Read the model definition and answer for the solid it produces. Units are mm, in the model's axes. Round coordinates to 2 decimals unless told otherwise and drop trailing zeros. Loops run counter-clockwise (first coordinate to the right, second up) from the corner with the lowest first, then second, coordinate; pieces in that order, holes last. Notation, with made-up numbers: (87.5, -25.5) -> (141.5, -25.5) arc R13 ccw to (141.5, -12.5) -> close; hole circle Ø5 at (24, 48.5). An arc over 180 degrees is marked (long way). Put each result on its own line as item: value.
from build123d import *

# Parameters (mm, degrees)
SKETCH1_W                     = 735.584
SKETCH1_H                     = 38.1
WOOD_BLOCK_DEPTH              = 19.05
SKETCH2_R                     = 7.9756
INNER_BORE_DEPTH              = 737.816349952
SKETCH3_R                     = 6.3881
MOUTHPIECE_THROUGH_HOLE_DEPTH = 737.816349952
SKETCH5_R                     = 8.128
COUNTERBORE_DEPTH             = 8.89
SKETCH4_OUTSIDE_W             = 187.464
SKETCH4_OUTSIDE_H             = 168.414
SKETCH4_OUTSIDE_R             = 14.2875
OUTER_DIAMETER_DEPTH          = 737.816350054


with BuildPart() as part:
    # Sketch1 → wood block (new body)
    with BuildSketch(Plane(origin=(0, 0, 0), x_dir=(1, 0, 0), z_dir=(0, 1, 0))):
        with Locations((367.792, 19.05)):
            Rectangle(SKETCH1_W, SKETCH1_H)
    extrude(amount=WOOD_BLOCK_DEPTH)

    # Sketch2 → inner bore (cut, through all)
    with BuildSketch(Plane(origin=(735.584, 0, 0), x_dir=(0, 0, -1), z_dir=(1, 0, 0))):
        with Locations((19.05, 19.05)):
            Circle(SKETCH2_R)
    extrude(amount=-INNER_BORE_DEPTH, mode=Mode.SUBTRACT)

    # Sketch3 → mouthpiece through hole (cut, through all)
    with BuildSketch(Plane(origin=(0, 0, 0), x_dir=(1, 0, 0), z_dir=(0, 1, 0))):
        with Locations(Location((22.225, 19.05, 0), (0, 0, 90))):
            Circle(SKETCH3_R)
    extrude(amount=MOUTHPIECE_THROUGH_HOLE_DEPTH, mode=Mode.SUBTRACT)

    # Sketch5 → counterbore (cut)
    with BuildSketch(Plane.XZ):
        with Locations(Location((22.225, -19.05, 0), (0, 0, 270))):
            Circle(SKETCH5_R)
        with Locations(Location((713.359, -19.05, 0), (0, 0, 90))):
            Circle(SKETCH5_R)
    extrude(amount=-COUNTERBORE_DEPTH, mode=Mode.SUBTRACT)

    # Sketch4 outside → outer diameter (cut, through all)
    with BuildSketch(Plane.ZY):
        with Locations((-19.05, 9.525)):
            Rectangle(SKETCH4_OUTSIDE_W, SKETCH4_OUTSIDE_H)
        with Locations((-19.05, 19.05)):
            Circle(SKETCH4_OUTSIDE_R, mode=Mode.SUBTRACT)
    extrude(amount=-OUTER_DIAMETER_DEPTH, mode=Mode.SUBTRACT)


solid = part.part
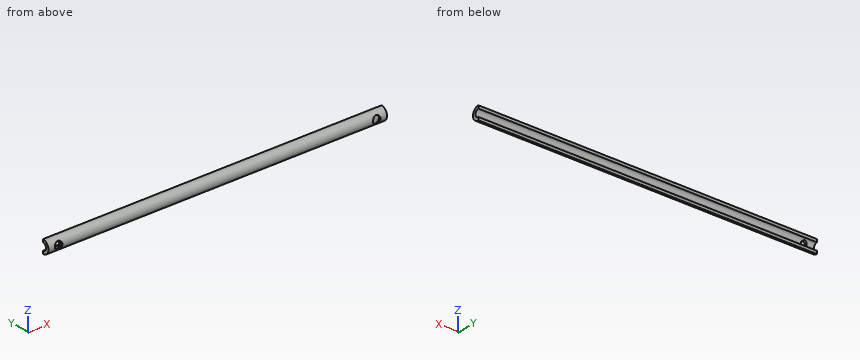
Item 1: The part is cut by section A-A (z = -19.05). Determine the outline of the cut face in (x, y), then the cut area to 3 significant figures.
Derived:
outline: (0, 4.76) -> (14.1, 4.76) -> (14.1, 8.89) -> (15.84, 8.89) -> (15.84, 11.07) -> (0, 11.07) -> close; (28.61, 8.89) -> (30.35, 8.89) -> (30.35, 4.76) -> (705.23, 4.76) -> (705.23, 8.89) -> (721.49, 8.89) -> (721.49, 4.76) -> (735.58, 4.76) -> (735.58, 11.07) -> (28.61, 11.07) -> close
area: 4,480 mm^2
Item 2: Find the intervals of material crossed by line 1 along X through (y, z) = (6.85, -19.05); line 2 along X through (y, z) = (5.5, -20); line 3 along X through (y, z) = (9.75, -20.25), in increasing order.
Derived:
line 1: x = 0 to 14.1, 30.35 to 705.23, 721.49 to 735.58
line 2: x = 0 to 14.15, 30.3 to 705.29, 721.43 to 735.58
line 3: x = 0 to 15.95, 28.5 to 735.58
Item 3: Flat-ended cylindrical pins translate along their axes: pin 1 Ø4 at (x, z) = (345.5, -11.5) entering from -Y; pin 2 Ø4 at (x, y) = (294, 15.5) entering from -Z; pin 3 Ø4 at (x, z) = (294.5, -13.5) entering from -Y. Find the tip coordinate at first contact, or state that the pin passes through.
Derived:
pin 1: stops at y = 5.88
pin 2: stops at z = -33.25
pin 3: stops at y = 5.21
